```python
from build123d import *

# Parameters (mm, degrees)
SKETCH_1_R          = 20
SKETCH_1_R_2        = 15.75
EXTRUDE_1_DEPTH     = 5
EXTRUDE_2_DEPTH     = 8
SKETCH_3_R          = 18
EXTRUDE_3_DEPTH     = 12
EXTRUDE_6_DEPTH     = 8
SKETCH_4_R          = 15
CUT_EXTRUDE_1_DEPTH = 16
SKETCH_7_R          = 2
CUT_EXTRUDE_2_DEPTH = 10
EXTRUDE_7_REACH     = 27
SKETCH_9_R          = 1.475
CUT_EXTRUDE_3_DEPTH = 5
SKETCH_10_W         = 1.475
SKETCH_10_H         = 47.880376143
SKETCH_11_W         = 47.783072431
SKETCH_11_H         = 1.475
SKETCH_12_R         = 2
CUT_EXTRUDE_4_DEPTH = 1.5


with BuildPart() as part:
    # 草图1 → 凸台-拉伸1 (new body)
    with BuildSketch(Plane.XY):
        Circle(SKETCH_1_R)
        Circle(SKETCH_1_R_2, mode=Mode.SUBTRACT)
    extrude(amount=EXTRUDE_1_DEPTH)

    # 草图2 → 凸台-拉伸2 (add)
    with BuildSketch(Plane.XY.offset(5)):
        with BuildLine():
            ThreePointArc((0, -25.892443989), (42.435244785, -24.5), (22.423514261, 12.946221995))
            ThreePointArc((22.423514261, 12.946221995), (0, 49), (-22.423514261, 12.946221995))
            ThreePointArc((-22.423514261, 12.946221995), (-42.435244785, -24.5), (0, -25.892443989))
        make_face()
    extrude(amount=EXTRUDE_2_DEPTH)

    # 草图3 → 凸台-拉伸3 (add)
    with BuildSketch(Plane.XY.offset(13)):
        with Locations((0, 42)):
            Circle(SKETCH_3_R)
        with Locations((36.373066959, -21)):
            Circle(SKETCH_3_R)
        with Locations((-36.373066959, -21)):
            Circle(SKETCH_3_R)
    extrude(amount=EXTRUDE_3_DEPTH)

    # 草图8 → 凸台-拉伸6 (add)
    with BuildSketch(Plane(origin=(0, 0, 5), x_dir=(-1, 0, 0), z_dir=(0, 0, -1))):
        with BuildLine():
            ThreePointArc((28.527895654, -41.553668461), (55.425625842, -32), (50.250480335, -3.929048123))
            ThreePointArc((50.250480335, -3.929048123), (31.431769398, 18.147140523), (21.72258468, 45.482716583))
            ThreePointArc((21.72258468, 45.482716583), (0, 64), (-21.72258468, 45.482716583))
            ThreePointArc((-21.72258468, 45.482716583), (-31.431769398, 18.147140523), (-50.250480335, -3.929048123))
            ThreePointArc((-50.250480335, -3.929048123), (-55.425625842, -32), (-28.527895654, -41.553668461))
            ThreePointArc((-28.527895654, -41.553668461), (0, -36.294281046), (28.527895654, -41.553668461))
        make_face()
        with BuildLine():
            ThreePointArc((22.423514261, 12.946221995), (42.435244785, -24.5), (0, -25.892443989))
            ThreePointArc((0, -25.892443989), (-42.435244785, -24.5), (-22.423514261, 12.946221995))
            ThreePointArc((-22.423514261, 12.946221995), (0, 49), (22.423514261, 12.946221995))
        make_face(mode=Mode.SUBTRACT)
    extrude(amount=-EXTRUDE_6_DEPTH)

    # 草图4 → 切除-拉伸1 (cut)
    with BuildSketch(Plane.XY.offset(25)):
        with Locations((0, 42)):
            Circle(SKETCH_4_R)
        with Locations((36.373066959, -21)):
            Circle(SKETCH_4_R)
        with Locations((-36.373066959, -21)):
            Circle(SKETCH_4_R)
    extrude(amount=-CUT_EXTRUDE_1_DEPTH, mode=Mode.SUBTRACT)

    # 草图7 → 切除-拉伸2 (cut)
    with BuildSketch(Plane.XY.offset(9)):
        with Locations((0, 42)):
            Circle(SKETCH_7_R)
        with Locations((36.373066959, -21)):
            Circle(SKETCH_7_R)
        with Locations((-36.373066959, -21)):
            Circle(SKETCH_7_R)
    extrude(amount=-CUT_EXTRUDE_2_DEPTH, mode=Mode.SUBTRACT)

    # 草图6 → 凸台-拉伸7 (add, up to next)
    with BuildSketch(Plane.XY.offset(25), mode=Mode.PRIVATE) as extrude_7_sk1:
        with BuildLine():
            ThreePointArc((2.644358031, 56.765072658), (0, 61.66268909), (-2.644358031, 56.765072658))
            ThreePointArc((-2.644358031, 56.765072658), (0, 57), (2.644358031, 56.765072658))
        make_face()
    extrude_7_tool1 = extrude(extrude_7_sk1.sketch, amount=-EXTRUDE_7_REACH, mode=Mode.PRIVATE) - part.part
    add(extrude_7_tool1.solids().sort_by_distance((0, 59.041522, 25))[0])
    # 草图6 → 凸台-拉伸7 (add, up to next)
    with BuildSketch(Plane.XY.offset(25), mode=Mode.PRIVATE) as extrude_7_sk2:
        with BuildLine():
            ThreePointArc((11.464748995, 32.327382439), (17.028388258, 32.168655455), (14.109107026, 36.907544902))
            ThreePointArc((14.109107026, 36.907544902), (12.990381057, 34.5), (11.464748995, 32.327382439))
        make_face()
    extrude_7_tool2 = extrude(extrude_7_sk2.sketch, amount=-EXTRUDE_7_REACH, mode=Mode.PRIVATE) - part.part
    add(extrude_7_tool2.solids().sort_by_distance((14.758391, 33.479239, 25))[0])
    # 草图6 → 凸台-拉伸7 (add, up to next)
    with BuildSketch(Plane.XY.offset(25), mode=Mode.PRIVATE) as extrude_7_sk3:
        with BuildLine():
            ThreePointArc((-14.109107026, 36.907544902), (-17.028388258, 32.168655455), (-11.464748995, 32.327382439))
            ThreePointArc((-11.464748995, 32.327382439), (-12.990381057, 34.5), (-14.109107026, 36.907544902))
        make_face()
    extrude_7_tool3 = extrude(extrude_7_sk3.sketch, amount=-EXTRUDE_7_REACH, mode=Mode.PRIVATE) - part.part
    add(extrude_7_tool3.solids().sort_by_distance((-14.758391, 33.479239, 25))[0])
    # 草图6 → 凸台-拉伸7 (add, up to next)
    with BuildSketch(Plane.XY.offset(25), mode=Mode.PRIVATE) as extrude_7_sk4:
        with BuildLine():
            ThreePointArc((47.837815954, -30.672617561), (53.401455217, -30.831344545), (50.482173985, -26.092455098))
            ThreePointArc((50.482173985, -26.092455098), (49.363448016, -28.5), (47.837815954, -30.672617561))
        make_face()
    extrude_7_tool4 = extrude(extrude_7_sk4.sketch, amount=-EXTRUDE_7_REACH, mode=Mode.PRIVATE) - part.part
    add(extrude_7_tool4.solids().sort_by_distance((51.131457, -29.520761, 25))[0])
    # 草图6 → 凸台-拉伸7 (add, up to next)
    with BuildSketch(Plane.XY.offset(25), mode=Mode.PRIVATE) as extrude_7_sk5:
        with BuildLine():
            ThreePointArc((22.263959933, -26.092455098), (19.344678701, -30.831344545), (24.908317964, -30.672617561))
            ThreePointArc((24.908317964, -30.672617561), (23.382685902, -28.5), (22.263959933, -26.092455098))
        make_face()
    extrude_7_tool5 = extrude(extrude_7_sk5.sketch, amount=-EXTRUDE_7_REACH, mode=Mode.PRIVATE) - part.part
    add(extrude_7_tool5.solids().sort_by_distance((21.614676, -29.520761, 25))[0])
    # 草图6 → 凸台-拉伸7 (add, up to next)
    with BuildSketch(Plane.XY.offset(25), mode=Mode.PRIVATE) as extrude_7_sk6:
        with BuildLine():
            ThreePointArc((39.01742499, -6.234927342), (36.373066959, -1.33731091), (33.728708928, -6.234927342))
            ThreePointArc((33.728708928, -6.234927342), (36.373066959, -6), (39.01742499, -6.234927342))
        make_face()
    extrude_7_tool6 = extrude(extrude_7_sk6.sketch, amount=-EXTRUDE_7_REACH, mode=Mode.PRIVATE) - part.part
    add(extrude_7_tool6.solids().sort_by_distance((36.373067, -3.958478, 25))[0])
    # 草图6 → 凸台-拉伸7 (add, up to next)
    with BuildSketch(Plane.XY.offset(25), mode=Mode.PRIVATE) as extrude_7_sk7:
        with BuildLine():
            ThreePointArc((-50.482173985, -26.092455098), (-53.401455217, -30.831344545), (-47.837815954, -30.672617561))
            ThreePointArc((-47.837815954, -30.672617561), (-49.363448016, -28.5), (-50.482173985, -26.092455098))
        make_face()
    extrude_7_tool7 = extrude(extrude_7_sk7.sketch, amount=-EXTRUDE_7_REACH, mode=Mode.PRIVATE) - part.part
    add(extrude_7_tool7.solids().sort_by_distance((-51.131457, -29.520761, 25))[0])
    # 草图6 → 凸台-拉伸7 (add, up to next)
    with BuildSketch(Plane.XY.offset(25), mode=Mode.PRIVATE) as extrude_7_sk8:
        with BuildLine():
            ThreePointArc((-33.728708928, -6.234927342), (-36.373066959, -1.33731091), (-39.01742499, -6.234927342))
            ThreePointArc((-39.01742499, -6.234927342), (-36.373066959, -6), (-33.728708928, -6.234927342))
        make_face()
    extrude_7_tool8 = extrude(extrude_7_sk8.sketch, amount=-EXTRUDE_7_REACH, mode=Mode.PRIVATE) - part.part
    add(extrude_7_tool8.solids().sort_by_distance((-36.373067, -3.958478, 25))[0])
    # 草图6 → 凸台-拉伸7 (add, up to next)
    with BuildSketch(Plane.XY.offset(25), mode=Mode.PRIVATE) as extrude_7_sk9:
        with BuildLine():
            ThreePointArc((-24.908317964, -30.672617561), (-19.344678701, -30.831344545), (-22.263959933, -26.092455098))
            ThreePointArc((-22.263959933, -26.092455098), (-23.382685902, -28.5), (-24.908317964, -30.672617561))
        make_face()
    extrude_7_tool9 = extrude(extrude_7_sk9.sketch, amount=-EXTRUDE_7_REACH, mode=Mode.PRIVATE) - part.part
    add(extrude_7_tool9.solids().sort_by_distance((-21.614676, -29.520761, 25))[0])

    # 草图9 → 切除-拉伸3 (cut)
    with BuildSketch(Plane.XY.offset(25)):
        with Locations((0, 59)):
            Circle(SKETCH_9_R)
        with Locations((14.722431864, 33.5)):
            Circle(SKETCH_9_R)
        with Locations((-14.722431864, 33.5)):
            Circle(SKETCH_9_R)
        with Locations((51.095498823, -29.5)):
            Circle(SKETCH_9_R)
        with Locations((21.650635095, -29.5)):
            Circle(SKETCH_9_R)
        with Locations((36.373066959, -4)):
            Circle(SKETCH_9_R)
        with Locations((-51.095498823, -29.5)):
            Circle(SKETCH_9_R)
        with Locations((-36.373066959, -4)):
            Circle(SKETCH_9_R)
        with Locations((-21.650635095, -29.5)):
            Circle(SKETCH_9_R)
    extrude(amount=-CUT_EXTRUDE_3_DEPTH, mode=Mode.SUBTRACT)

    # 草图10 → 切除-旋转1 (revolve, cut)
    with BuildSketch(Plane(origin=(0, 0, 2.5), x_dir=(-1, 0, 0), z_dir=(0, 0, -1))):
        with Locations((0.7375, -0.269128361)):
            Rectangle(SKETCH_10_W, SKETCH_10_H)
    revolve(axis=Axis((0, 26.597082696, 2.5), (0, -1, 0)), mode=Mode.SUBTRACT)

    # 草图11 → 切除-旋转2 (revolve, cut)
    with BuildSketch(Plane(origin=(0, 0, 2.5), x_dir=(-1, 0, 0), z_dir=(0, 0, -1))):
        with Locations((0.227220258, 0.7375)):
            Rectangle(SKETCH_11_W, SKETCH_11_H)
    revolve(axis=Axis((35.344622551, 0, 2.5), (-1, 0, 0)), mode=Mode.SUBTRACT)

    # 草图12 → 切除-拉伸4 (cut)
    with BuildSketch(Plane(origin=(0, 0, 5), x_dir=(-1, 0, 0), z_dir=(0, 0, -1))):
        Polygon((-6.5, 32), (0, 32), (6.5, 32), (6.5, 60), (-6.5, 60), align=None)
        with Locations((0, 42)):
            Circle(SKETCH_12_R, mode=Mode.SUBTRACT)
        Polygon((-30.962812921, -10.370834875), (-55.211524227, -24.370834875), (-48.711524227, -35.629165125), (-24.462812921, -21.629165125), (-27.712812921, -16), align=None)
        with Locations((-36.373066959, -21)):
            Circle(SKETCH_12_R, mode=Mode.SUBTRACT)
        Polygon((24.462812921, -21.629165125), (48.711524227, -35.629165125), (55.211524227, -24.370834875), (30.962812921, -10.370834875), (27.712812921, -16), align=None)
        with Locations((36.373066959, -21)):
            Circle(SKETCH_12_R, mode=Mode.SUBTRACT)
    extrude(amount=-CUT_EXTRUDE_4_DEPTH, mode=Mode.SUBTRACT)


solid = part.part
```
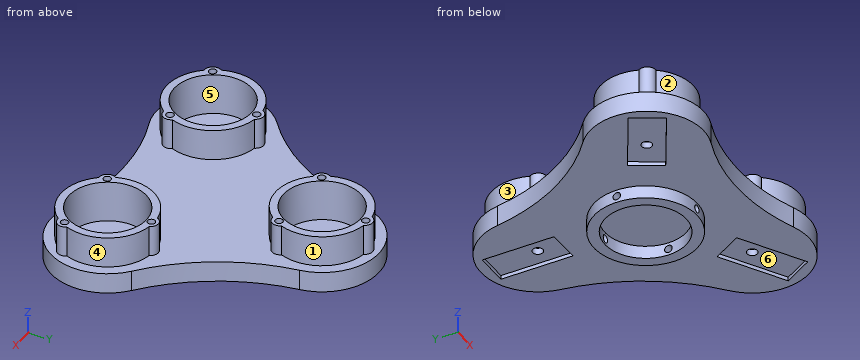
Geometry: final body of the model. Coordinates: model frame, mm. Face numbers are marked on the shaded views. A direction names the side the tool comes from. Coordinates: 2 decimals unless noted, no trailing zeros. Order: outer loops, then holes, each group sorted by start corner. A loop starts at its lowest first (then second) coordinate and runs counter-clockwise, first axis right, second up. Notation, with made-up numbers: (-31.5, 28.5) -> (-18.5, 28.5) arc R29 ccw to (-18.5, 57.5) -> close; hole circle Ø5 at (4, -6.75). An arc over 180 degrees is marked (long way). Use CSV: the item, a comma, the result in double quotes.
1) Access query for the marked faces 4, 5 and 6. Directions: +Z, -Z, +X, -X, +Y, -Y. A direction counts if a zero-diameter tool reaches every point of the face in a straight line with its end or side. Return the directions, or none.
Findings:
face 4,"+Z, +X"
face 5,"+Z"
face 6,"-Z"
2) Section A-A on z = 15. Output: boundary loops of the cut face in (x, y), then the cut area to 3 significant figures.
Findings:
outline,"(-53.21, -27.37) arc R3.16 ccw to (-50.31, -32.39) arc R18 ccw to (-22.44, -32.39) arc R3.16 ccw to (-19.54, -27.37) arc R18 ccw to (-33.47, -3.23) arc R3.16 ccw to (-39.27, -3.23) arc R18 ccw to start; (-16.83, 35.63) arc R3.16 ccw to (-13.94, 30.61) arc R18 ccw to (13.94, 30.61) arc R3.16 ccw to (16.83, 35.63) arc R18 ccw to (2.9, 59.77) arc R3.16 ccw to (-2.9, 59.77) arc R18 ccw to start; (19.54, -27.37) arc R3.16 ccw to (22.44, -32.39) arc R18 ccw to (50.31, -32.39) arc R3.16 ccw to (53.21, -27.37) arc R18 ccw to (39.27, -3.23) arc R3.16 ccw to (33.47, -3.23) arc R18 ccw to start; hole circle Ø30 at (-36.37, -21); hole circle Ø30 at (0, 42); hole circle Ø30 at (36.37, -21)"
area,"996 mm^2"
3) Mould query, pull axis X, two halves, no side actions, for the marked faces 1, 2 and 3. Classes: +X half, -X half, draft (parallel to the pull), parting line (faces both ways), or undercut.
Findings:
face 1,"+X half"
face 2,"undercut"
face 3,"-X half"
4) Line query: line 1 (Z direction, x = 0, y = -16.8) (3 decimals); line 2 (X direction, y = -9.5, z = 24.25); line 3 (X direction, y = -19, z = 16.5). Output: solid intervals per line, ascending.
Findings:
line 1,"z = 0 to 1.025, 3.975 to 13"
line 2,"x = -50.22 to -46, -26.74 to -22.53, 22.53 to 26.74, 46 to 50.22"
line 3,"x = -54.26 to -51.24, -21.51 to -18.48, 18.48 to 21.51, 51.24 to 54.26"
5) Pin query (flat end, axial travel): pin 1 Ø2.5 at (x, y) = (36.37, -4) entering from +Z; pin 2 Ø15 at (x, y) = (33.5, -17) entering from +Z; pin 3 Ø1.5 at (x, y) = (-1, -14.5) entering from -Z. Return the tip coordinate at first contact, or that it passes through.
Findings:
pin 1,"stops at z = 20"
pin 2,"stops at z = 9"
pin 3,"stops at z = 5"
6) Section B-B on y = 42. Output: boundary loops of the cut face in (x, z).
Findings:
outline,"(-22.36, 5) -> (-6.5, 5) -> (-6.5, 6.5) -> (-2, 6.5) -> (-2, 9) -> (-15, 9) -> (-15, 25) -> (-18, 25) -> (-18, 13) -> (-22.36, 13) -> close; (2, 6.5) -> (6.5, 6.5) -> (6.5, 5) -> (22.36, 5) -> (22.36, 13) -> (18, 13) -> (18, 25) -> (15, 25) -> (15, 9) -> (2, 9) -> close"
7) Section C-C on z = 2.5. Output: boundary loops of the cut face in (x, y) (3 decimals).
Findings:
outline,"(-19.946, -1.475) arc R20 ccw to (-1.475, -19.946) -> (-1.475, -15.681) arc R15.75 cw to (-15.681, -1.475) -> close; (-19.946, 1.475) -> (-15.681, 1.475) arc R15.75 cw to (-1.475, 15.681) -> (-1.475, 19.946) arc R20 ccw to start; (1.475, -19.946) arc R20 ccw to (19.946, -1.475) -> (15.681, -1.475) arc R15.75 cw to (1.475, -15.681) -> close; (1.475, 15.681) arc R15.75 cw to (15.681, 1.475) -> (19.946, 1.475) arc R20 ccw to (1.475, 19.946) -> close"
8) Section D-D on y = 0. Output: boundary loops of the cut face in (x, z) (3 decimals), then the cut area to 3 significant figures.
Findings:
outline,"(-45.769, 5) -> (-20, 5) -> (-20, 3.975) -> (-15.75, 3.975) -> (-15.75, 5) -> (15.75, 5) -> (15.75, 3.975) -> (20, 3.975) -> (20, 5) -> (45.769, 5) -> (45.769, 13) -> (-45.769, 13) -> close; (-20, 0) -> (-15.75, 0) -> (-15.75, 1.025) -> (-20, 1.025) -> close; (15.75, 0) -> (20, 0) -> (20, 1.025) -> (15.75, 1.025) -> close"
area,"750 mm^2"
